Geometry check sheet. Reference: the model listing, model coordinates, mm. A direction names the side the tool comes from. Give positions to 0.01 mm unless a question says otherwise; leave off trailing zeros. Order: outer loops, then holes, each group sorted by start corner. A loop starts at its lowest first (then second) coordinate and runs counter-clockwise, first axis right, second up. Notation, with made-up numbers: M 42,55.5 L 46,55.5 A7 cw 46,61.5 Z; hole C -19,-7 d7. An arc over 180 degrees is marked long. Answer as a JSON object with one key per item and string values. Group by question number.
from build123d import *

# Parameters (mm, degrees)
SKETCH1_R                   = 19.05
BOSS_EXTRUDE1_DEPTH         = 12.7
FILLET1_R                   = 25.4
FILLET2_R                   = 50.8
F_1_2_CLEARANCE_HOLE1_D     = 13.49248
F_1_2_CLEARANCE_HOLE1_DEPTH = 38.1
F_1_2_CLEARANCE_HOLE1_TIP   = 4.053549943
SKETCH4_R                   = 19.05
CUT_EXTRUDE1_DEPTH          = 13.7
BOSS_EXTRUDE2_DEPTH         = 12.7
FILLET3_R                   = 19.05
FILLET4_R                   = 50.8
BOSS_EXTRUDE3_DEPTH         = 12.7
CUT_EXTRUDE2_DEPTH          = 13.7
FILLET7_R                   = 6.35


with BuildPart() as part:
    # Sketch1 → Boss-Extrude1 (new body)
    with BuildSketch(Plane(origin=(0, 0, 0), x_dir=(0, 0, -1), z_dir=(1, 0, 0))):
        with BuildLine():
            Line((390.630407277, -109.766978243), (305.29908743, -24.435658396))
            Line((305.29908743, -24.435658396), (12.395871839, 49.264412727))
            ThreePointArc((12.395871839, 49.264412727), (-49.470959365, 11.544010545), (-10.688712274, -49.662777107))
            Line((-10.688712274, -49.662777107), (281.610658396, -75.235658396))
            Line((281.610658396, -75.235658396), (339.725, -133.35))
            Line((339.725, -133.35), (339.725, -254))
            Line((339.725, -254), (390.630407277, -254))
            Line((390.630407277, -254), (390.630407277, -109.766978243))
        make_face()
        Circle(SKETCH1_R, mode=Mode.SUBTRACT)
    extrude(amount=BOSS_EXTRUDE1_DEPTH)

    # Fillet1
    fillet1_edges = [part.edges().sort_by_distance(p)[0] for p in [
        (6.35, -133.35, -339.725),
        (6.35, -75.235658396, -281.610658396),
    ]]
    fillet(fillet1_edges, radius=FILLET1_R)

    # Fillet2
    fillet2_edges = [part.edges().sort_by_distance(p)[0] for p in [
        (6.35, -24.435658396, -305.29908743),
        (6.35, -109.766978243, -390.630407277),
    ]]
    fillet(fillet2_edges, radius=FILLET2_R)

    # 1/2 Clearance Hole1
    with Locations(Plane(origin=(12.7, 0, 0), x_dir=(0, 0, -1), z_dir=(1, 0, 0))):
        with Locations((365.125, -234.95), (365.125, -196.85), (365.125, -158.75), (359.5071206, -120.65), (324.846024484, -82.55)):
            Hole(F_1_2_CLEARANCE_HOLE1_D / 2, depth=F_1_2_CLEARANCE_HOLE1_DEPTH)
            with Locations((0, 0, -(F_1_2_CLEARANCE_HOLE1_DEPTH + F_1_2_CLEARANCE_HOLE1_TIP / 2))):  # 118° drill point
                Cone(0, F_1_2_CLEARANCE_HOLE1_D / 2, F_1_2_CLEARANCE_HOLE1_TIP, mode=Mode.SUBTRACT)

    # Sketch4 → Cut-Extrude1 (cut, through all)
    with BuildSketch(Plane(origin=(12.7, 0, 0), x_dir=(0, 0, -1), z_dir=(1, 0, 0))):
        with BuildLine():
            Line((288.147750244, -81.772750244), (306.885512242, -100.510512242))
            ThreePointArc((306.885512242, -100.510512242), (306.885512242, -63.266297725), (344.129726759, -63.266297725))
            Line((344.129726759, -63.266297725), (315.219181895, -34.355752861))
            ThreePointArc((315.219181895, -34.355752861), (304.360921026, -26.089699144), (291.69402925, -21.012364618))
            Line((291.69402925, -21.012364618), (12.395871839, 49.264412727))
            ThreePointArc((12.395871839, 49.264412727), (-49.470959365, 11.544010545), (-10.688712274, -49.662777107))
            Line((-10.688712274, -49.662777107), (272.400993868, -74.429917155))
            ThreePointArc((272.400993868, -74.429917155), (280.92174185, -76.713044696), (288.147750244, -81.772750244))
        make_face()
        Circle(SKETCH4_R, mode=Mode.SUBTRACT)
    extrude(amount=-CUT_EXTRUDE1_DEPTH, mode=Mode.SUBTRACT)

    # Sketch5 → Boss-Extrude2 (add)
    with BuildSketch(Plane(origin=(12.7, 0, 0), x_dir=(0, 0, -1), z_dir=(1, 0, 0))):
        Polygon((339.725, -254), (390.630407277, -260.723431786), (762, -260.723431786), (673.1, -209.923431786), (679.45, -228.973431786), (607.332959214, -219.448431786), (610.507959214, -228.973431786), (538.390918427, -219.448431786), (541.565918427, -228.973431786), (469.448877641, -219.448431786), (472.623877641, -228.973431786), (400.506836855, -219.448431786), (390.630407277, -218.143982925), (390.630407277, -254), align=None)
    extrude(amount=-BOSS_EXTRUDE2_DEPTH)

    # Fillet3
    fillet3_edges = [part.edges().sort_by_distance(p)[0] for p in [
        (6.35, -260.723431786, -390.630407277),
        (6.35, -254, -339.725),
    ]]
    fillet(fillet3_edges, radius=FILLET3_R)

    # Fillet4
    fillet4_edges = [part.edges().sort_by_distance(p)[0] for p in [
        (6.35, -218.143982925, -390.630407277),
    ]]
    fillet(fillet4_edges, radius=FILLET4_R)

    # Sketch6 → Boss-Extrude3 (add)
    with BuildSketch(Plane(origin=(12.7, 0, 0), x_dir=(0, 0, -1), z_dir=(1, 0, 0))):
        with BuildLine():
            Line((375.751431761, -94.888002727), (344.129726759, -63.266297725))
            Line((344.129726759, -63.266297725), (309.842868861, -60.718111058))
            ThreePointArc((309.842868861, -60.718111058), (398.793863401, -27.03548328), (492.230407277, -44.823431786))
            ThreePointArc((492.230407277, -44.823431786), (421.492844328, -64.2581395), (390.630407277, -130.809027211))
            Line((390.630407277, -130.809027211), (375.751431761, -94.888002727))
        make_face()
    extrude(amount=-BOSS_EXTRUDE3_DEPTH)

    # Sketch7 → Cut-Extrude2 (cut, through all)
    with BuildSketch(Plane(origin=(12.7, 0, 0), x_dir=(0, 0, -1), z_dir=(1, 0, 0))):
        with BuildLine():
            Line((338.534408325, -57.67097929), (375.751431761, -94.888002727))
            ThreePointArc((375.751431761, -94.888002727), (379.072218132, -98.54883067), (382.021527149, -102.515045449))
            ThreePointArc((382.021527149, -102.515045449), (401.979554881, -65.801657117), (435.210476685, -40.465880242))
            ThreePointArc((435.210476685, -40.465880242), (385.540929372, -41.58660974), (338.534408325, -57.67097929))
        make_face()
    extrude(amount=-CUT_EXTRUDE2_DEPTH, mode=Mode.SUBTRACT)

    # Fillet7
    fillet7_edges = [part.edges().sort_by_distance(p)[0] for p in [
        (6.35, -102.515045449, -382.021527149),
        (6.35, -40.465880242, -435.210476685),
        (6.35, -57.67097929, -338.534408325),
    ]]
    fillet(fillet7_edges, radius=FILLET7_R)


solid = part.part
1. Thickness scan on line 1 along Y through (x, z) = (5, -360.5); line 2 along Z through (x, y) = (12, -83.5); line 3 along Z through (x, y) = (9, -79). Record the ranges inside material, lowest first. Write a range as [from, to].
2. Cross-section at A-A (y = -158.75). Record the cut outline in (x, z) (3 decimals), and give its area (3 significant figures).
3. Cross-section at C-C (y = -120.65). Record the cut outline in (x, z) (3 decimals).
4. Cross-section at D-D (x = 4.25). State how many separate pieces and enclosed holes the cut face has, and give its area (3 significant figures).
5. Access from +Z, -Z, +X, -X, +Y, -Y to the whole of each face (thin tool, end or side, straight path). Record for faces 1 (the cylindrical face through (6.261, -58.418, -343.044)), 2 (the flat face through (6, -153, -390.63)), 3 (the flat face through (6.261, -113.033, -319.408)).
6. Depth check by flat-ended pin: pin 1 (2 mm diameter, centred on x = 2, y = -106.5, fed in from +Z) (3 decimals); pin 2 (1.5 mm diameter, centred on x = 3, y = -140, fed in from -Z); pin 3 (11 mm diameter, centred on y = -82.55, z = -324.85, fed in from +X); pin 4 (6 mm diameter, centred on x = 6.5, y = -66, fed in from +Z). Enter the tip coordinate at first touch or a pass-through.
7. Cross-section at B-B (y = -82.55). Record the cut outline in (x, z).
Report:
{
 "1": {"line 1": "y = [-256.74, -239.86], [-230.04, -201.76], [-191.94, -163.66], [-153.84, -127.32], [-113.98, -79.64], [-48.14, -34.75]", "line 2": "z = [-404.58, -389.84], [-364.36, -331.53], [-318.17, -299.22]", "line 3": "z = [-407.69, -392.42], [-359.86, -330.58], [-319.11, -299.33]"},
 "2": {"outline": "M 0,-390.63 L 12.7,-390.63 L 12.7,-371.871 L 0,-371.871 Z; M 0,-358.379 L 12.7,-358.379 L 12.7,-339.725 L 0,-339.725 Z", "area": "475 mm2"},
 "3": {"outline": "M 0,-391.224 L 12.7,-391.224 L 12.7,-366.253 L 0,-366.253 Z; M 0,-352.761 L 12.7,-352.761 L 12.7,-327.025 L 0,-327.025 Z"},
 "4": {"separate pieces": "1", "enclosed holes": "6", "area": "26,400 mm2"},
 "5": {"face 1": "+X, -X", "face 2": "-Z, +X, -X", "face 3": "+Z, +X, -X, -Y"},
 "6": {"pin 1": "stops at z = -311.875", "pin 2": "stops at z = -390.63", "pin 3": "passes through", "pin 4": "stops at z = -302.54"},
 "7": {"outline": "M 0,-405.2 L 12.7,-405.2 L 12.7,-390.36 L 0,-390.36 Z; M 0,-363.41 L 12.7,-363.41 L 12.7,-331.59 L 0,-331.59 Z; M 0,-318.1 L 12.7,-318.1 L 12.7,-299.18 L 0,-299.18 Z"}
}
